```python
from build123d import *

# Parameters (mm, degrees)
F1_DEPTH        = 5
F4_DEPTH        = 13.5
F6_DEPTH        = 7.5
F8_DEPTH        = 6.5
F10_D           = 3
F10_CSINK_D     = 7.5
F10_CSINK_ANGLE = 90
F12_D           = 2
F12_CSINK_D     = 5
F12_CSINK_ANGLE = 90


with BuildPart() as f1:
    # F0 (on Front) → F1 (new body)
    with BuildSketch(Plane.XZ):
        Polygon((19.12546, 114.327021), (-0.37454, 114.327021), (-0.37454, -0.672979), (19.62546, -0.672979), (19.62546, 29.327021), (13.12546, 29.327021), (13.12546, 39.827021), (5.62546, 39.827021), (5.62546, 48.327021), (19.12546, 48.327021), (19.12546, 75.827021), (5.62546, 75.827021), (5.62546, 84.327021), (19.12546, 84.327021), align=None)
    extrude(amount=F1_DEPTH)

    # F2 (on face) + F3 (on face) → F4 (cut)
    with BuildSketch(Plane.YZ.offset(19.12546)):
        Polygon((0, 89.327021), (-5, 84.327021), (0, 84.327021), align=None)
    with BuildSketch(Plane.YZ.offset(19.12546)):
        Polygon((-5, 70.827021), (0, 75.827021), (-5, 75.827021), align=None)
        Polygon((-5, 48.327021), (0, 48.327021), (-5, 53.327021), align=None)
    extrude(amount=-F4_DEPTH, mode=Mode.SUBTRACT)

    # F5 (on face) → F6 (cut)
    with BuildSketch(Plane.YZ.offset(13.12546)):
        Polygon((0, 39.827021), (-5, 39.827021), (0, 34.827021), align=None)
    extrude(amount=-F6_DEPTH, mode=Mode.SUBTRACT)

    # F7 (on face) → F8 (cut)
    with BuildSketch(Plane.YZ.offset(19.62546)):
        Polygon((-5, 24.327021), (0, 29.327021), (-5, 29.327021), align=None)
    extrude(amount=-F8_DEPTH, mode=Mode.SUBTRACT)

    # F10 (through all)
    with Locations(Plane(origin=(0, 0, 0), x_dir=(-1, 0, 0), z_dir=(0, 1, 0))):
        with Locations((-12.37546, 105.327021), (-12.37546, 8.327021)):
            CounterSinkHole(F10_D / 2, F10_CSINK_D / 2, counter_sink_angle=F10_CSINK_ANGLE)

    # F12 (through all)
    with Locations(Plane.XZ.offset(5)):
        with Locations((2.62546, 11.827021), (2.62546, 99.327021)):
            CounterSinkHole(F12_D / 2, F12_CSINK_D / 2, counter_sink_angle=F12_CSINK_ANGLE)


solid = f1.part
```
Check sheet for the modelled part. Datum: model origin and axes. Units: mm. A direction names the side the tool comes from. Round coordinates to 2 decimals unless told otherwise and drop trailing zeros. Loops run counter-clockwise (first coordinate to the right, second up) from the corner with the lowest first, then second, coordinate; pieces in that order, holes last. Notation, with made-up numbers: (38, -25.75) - (58, -25.75) arc R19 cw to (58, 11.25) - close; hole circle Ø11 at (33, 70.5). An arc over 180 degrees is marked (long way). Answer as a JSON object with one key per item and string values. Group by question number.
Q1. Set-up check for faces 5 (the face through (12.47, -2.465, 86.862)), 6 (the face through (19.125, -2, 62)), 7 (the face through (16.421, -2.535, 26.792)): record each of +Z, -Z, +X, -X, +Y, -Y from which the full face is reachable in a straight line by a thin tool's end or side.
Q2. Scan lines: line 1 along Z through (x, y) = (16.25, -3.2); line 2 along Z through (x, y) = (19, -4.7); line 3 along X through (y, z) = (-2.8, 99). Record each from-to range of solid material in increasing order. Write a range as [from, to].
Q3. Sectioned sample at A-A, the plane y = -1. Enter the section's corners in (x, z), plus the area to 3 significant figures.
Q4. Mould release check, pull along Z, two halves, no side actions. Record for faces 1 (the face through (10.877, -3.644, 8.393)), 2 (the face through (7, 0, 58)), 3 (the face through (10.768, -2.141, 8.398)), 4 (the face through (10, -2, 114.327)): released by +Z, released by -Z, zero draft, split by the parting line, or undercut.
Q5. Sectioned sample at C-C, the plane x = 12. Count the separate pieces of the cut face and the enclosed holes in it, plus the area to 3 significant figures.
Q6. Gauge pin test, flat ends, axial feed: P1, Ø3, axis at x = 2.63, z = 99.33, coming from the +Y side; P2, Ø1.5, axis at y = -3, z = 57, coming from the +X side; P3, Ø2.5, axis at x = 12.38, z = 8.33, coming from the -Y side; P4, Ø2.5, axis at y = -3.5, z = 28.5, coming from the +X side. Record the tip position at first contact, or that the pin passes through.
Q7. Sectioned sample at B-B, the plane z = 47. Enter the section's corners in (x, y).
Q8. Sectioned sample at D-D, the plane z = 74. Enter the section's corners in (x, y), plus the area to 3 significant figures.
Solution:
{
 "1": {"face 5": "+X, +Y", "face 6": "+Z, +X, +Y, -Y", "face 7": "+X, -Y"},
 "2": {"line 1": "z = [-0.67, 26.13], [51.53, 72.63], [86.13, 114.33]", "line 2": "z = [-0.67, 24.63], [53.03, 71.13], [84.63, 114.33]", "line 3": "x = [-0.37, 1.68], [3.57, 19.13]"},
 "3": {"outline": "(-0.37, -0.67) - (19.63, -0.67) - (19.63, 28.33) - (13.13, 28.33) - (13.13, 35.83) - (5.63, 35.83) - (5.63, 49.33) - (19.13, 49.33) - (19.13, 74.83) - (5.63, 74.83) - (5.63, 88.33) - (19.13, 88.33) - (19.13, 114.33) - (-0.37, 114.33) - close; hole circle Ø2 at (2.63, 11.83); hole circle Ø2 at (2.63, 99.33); hole circle Ø5.5 at (12.38, 8.33); hole circle Ø5.5 at (12.38, 105.33)", "area": "1,790 mm²"},
 "4": {"face 1": "undercut", "face 2": "zero draft", "face 3": "undercut", "face 4": "released by +Z"},
 "5": {"separate pieces": "5", "enclosed holes": "0", "area": "401 mm²"},
 "6": {"P1": "stops at y = 0", "P2": "stops at x = 19.13", "P3": "passes through", "P4": "stops at x = 13.13"},
 "7": {"outline": "(-0.37, -5) - (5.63, -5) - (5.63, 0) - (-0.37, 0) - close"},
 "8": {"outline": "(-0.37, -5) - (5.63, -5) - (5.63, -1.83) - (19.13, -1.83) - (19.13, 0) - (-0.37, 0) - close", "area": "54.7 mm²"}
}
